from build123d import *

# Parameters (mm, degrees)
BOSS_EXTRUDE1_DEPTH = 16
SKETCH2_W           = 1.5
SKETCH2_H           = 16
BOSS_EXTRUDE2_DEPTH = 0.8
SKETCH3_W           = 16.5
SKETCH3_H           = 16
BOSS_EXTRUDE3_DEPTH = 20.8
SKETCH4_W           = 24.15
SKETCH4_H           = 16
BOSS_EXTRUDE4_DEPTH = 3.5
CUT_EXTRUDE1_DEPTH  = 6.5
CUT_EXTRUDE2_DEPTH  = 2
CUT_EXTRUDE3_DEPTH  = 2
SKETCH8_W           = 3
SKETCH8_H           = 7
CUT_EXTRUDE4_DEPTH  = 2.5
CUT_EXTRUDE5_DEPTH  = 1
SKETCH10_W          = 3.5
SKETCH10_H          = 16
BOSS_EXTRUDE5_DEPTH = 1.85
SKETCH11_W          = 2
SKETCH11_H          = 16.5
CUT_EXTRUDE6_DEPTH  = 9.8
SKETCH12_W          = 16.5
SKETCH12_H          = 1
CUT_EXTRUDE7_DEPTH  = 5.5
BOSS_EXTRUDE6_DEPTH = 7.5
CUT_EXTRUDE8_DEPTH  = 7.5
CUT_EXTRUDE9_DEPTH  = 7.5
SKETCH16_W          = 0.6
SKETCH16_H          = 7
BOSS_EXTRUDE7_DEPTH = 8
SKETCH17_W          = 6.5
SKETCH17_H          = 1.1
CUT_EXTRUDE10_DEPTH = 33.205641493
SKETCH18_W          = 6.5
SKETCH18_H          = 1.1
CUT_EXTRUDE11_DEPTH = 33.205641493
SKETCH19_W          = 0.6
SKETCH19_H          = 7
BOSS_EXTRUDE8_DEPTH = 8
SKETCH20_W          = 6.5
SKETCH20_H          = 1.1
CUT_EXTRUDE12_DEPTH = 32.849473214
SKETCH21_W          = 6.5
SKETCH21_H          = 1.1
CUT_EXTRUDE13_DEPTH = 32.849473214
CUT_EXTRUDE14_REACH = 33.068
CUT_EXTRUDE15_REACH = 34.206
CUT_EXTRUDE16_DEPTH = 32.849473214
CUT_EXTRUDE17_DEPTH = 7.5
CUT_EXTRUDE18_DEPTH = 1.5
CUT_EXTRUDE19_DEPTH = 1.5
SKETCH28_W          = 1.524
SKETCH28_H          = 7.988
CUT_EXTRUDE20_DEPTH = 18
SKETCH29_W          = 1.524
SKETCH29_H          = 6.35
CUT_EXTRUDE21_DEPTH = 18
CHAMFER1_SIZE       = 0.5
CHAMFER2_SIZE       = 0.528136002
CHAMFER2_SIZE2      = 0.608008164
CHAMFER3_SIZE       = 0.4
CHAMFER3_SIZE2      = 0.692820323
CHAMFER4_SIZE       = 0.608008164
CHAMFER4_SIZE2      = 0.528136002
CHAMFER5_SIZE       = 1.5
CHAMFER5_SIZE2      = 2.598076211


with BuildPart() as part:
    # Sketch1 → Boss-Extrude1 (new body)
    with BuildSketch(Plane.XZ.offset(8)):
        Polygon((12.803267754, -0.8), (9.65, -0.8), (9.65, -14.690909091), (10.15, -11.6), (10.15, -8.6), align=None)
    extrude(amount=-BOSS_EXTRUDE1_DEPTH)

    # Sketch2 → Boss-Extrude2 (add)
    with BuildSketch(Plane.XY.offset(-0.8)):
        with Locations((10.4, 0)):
            Rectangle(SKETCH2_W, SKETCH2_H)
    extrude(amount=BOSS_EXTRUDE2_DEPTH)

    # Sketch3 → Boss-Extrude3 (add)
    with BuildSketch(Plane.ZY.offset(-9.65)):
        with Locations((-8.25, 0)):
            Rectangle(SKETCH3_W, SKETCH3_H)
    extrude(amount=BOSS_EXTRUDE3_DEPTH)

    # Sketch4 → Boss-Extrude4 (add)
    with BuildSketch(Plane.XY):
        with Locations((0.925, 0)):
            Rectangle(SKETCH4_W, SKETCH4_H)
    extrude(amount=BOSS_EXTRUDE4_DEPTH)

    # Sketch5 → Cut-Extrude1 (cut)
    with BuildSketch(Plane(origin=(0, 8, 0), x_dir=(-1, 0, 0), z_dir=(0, 1, 0))):
        Polygon((-9.65, -14.690909091), (-9.65, -6.5), (-11.15, -3.5), (-11.15, -0.8), (-12.803267754, -0.8), (-10.15, -8.6), (-10.15, -11.6), align=None)
    extrude(amount=-CUT_EXTRUDE1_DEPTH, mode=Mode.SUBTRACT)

    # Sketch6 → Cut-Extrude2 (cut)
    with BuildSketch(Plane(origin=(0, 8, 0), x_dir=(-1, 0, 0), z_dir=(0, 1, 0))):
        Polygon((-11.15, 0), (-11.15, -3.5), (-9.65, -6.5), (-9.65, -16.5), (11.15, -16.5), (11.15, 0), align=None)
    extrude(amount=-CUT_EXTRUDE2_DEPTH, mode=Mode.SUBTRACT)

    # Sketch7 → Cut-Extrude3 (cut)
    with BuildSketch(Plane.XZ.offset(8)):
        Polygon((11.15, -0.8), (11.15, 0), (-11.15, 0), (-11.15, -16.5), (9.65, -16.5), (9.65, -14.690909091), (10.15, -11.6), (10.15, -8.6), (12.803267754, -0.8), align=None)
    extrude(amount=-CUT_EXTRUDE3_DEPTH, mode=Mode.SUBTRACT)

    # Sketch8 → Cut-Extrude4 (cut)
    with BuildSketch(Plane.XZ.offset(6)):
        with Locations((0, -3.5)):
            Rectangle(SKETCH8_W, SKETCH8_H)
    extrude(amount=-CUT_EXTRUDE4_DEPTH, mode=Mode.SUBTRACT)

    # Sketch9 → Cut-Extrude5 (cut)
    with BuildSketch(Plane.XZ.offset(6)):
        Polygon((-1.5, -7), (-1.5, -16.5), (7, -16.5), (7, 0), (1.5, 0), (1.5, -7), align=None)
    extrude(amount=-CUT_EXTRUDE5_DEPTH, mode=Mode.SUBTRACT)

    # Sketch10 → Boss-Extrude5 (add)
    with BuildSketch(Plane.ZY.offset(11.15)):
        with Locations((1.75, 0)):
            Rectangle(SKETCH10_W, SKETCH10_H)
    extrude(amount=BOSS_EXTRUDE5_DEPTH)

    # Sketch11 → Cut-Extrude6 (cut)
    with BuildSketch(Plane.XZ.offset(6)):
        with Locations((-10.15, -8.25)):
            Rectangle(SKETCH11_W, SKETCH11_H)
    extrude(amount=-CUT_EXTRUDE6_DEPTH, mode=Mode.SUBTRACT)

    # Sketch12 → Cut-Extrude7 (cut)
    with BuildSketch(Plane(origin=(-1.5, 0, 0), x_dir=(0, 0, -1), z_dir=(1, 0, 0))):
        with Locations((8.25, -5.5)):
            Rectangle(SKETCH12_W, SKETCH12_H)
    extrude(amount=-CUT_EXTRUDE7_DEPTH, mode=Mode.SUBTRACT)

    # Sketch13 → Boss-Extrude6 (add)
    with BuildSketch(Plane.XZ.offset(6)):
        Polygon((-9.15, -6.566987298), (-10.695259589, -0.8), (-12.803267754, -0.8), (-10.15, -8.6), (-10.15, -11.6), (-9.6, -15), (-9.6, -16.5), (-9.15, -16.5), align=None)
    extrude(amount=-BOSS_EXTRUDE6_DEPTH)

    # Sketch14 → Cut-Extrude8 (cut)
    with BuildSketch(Plane.XZ.offset(6)):
        with BuildLine():
            Line((-9.15, 0), (-9.15, -6.566987298))
            Line((-9.15, -6.566987298), (-8.9, -7.5))
            Line((-8.9, -7.5), (-8.9, -9.5))
            ThreePointArc((-8.9, -9.5), (-8.45, -9.95), (-8, -9.5))
            Line((-8, -9.5), (-8, 0))
            Line((-8, 0), (-9.15, 0))
        make_face()
    extrude(amount=-CUT_EXTRUDE8_DEPTH, mode=Mode.SUBTRACT)

    # Sketch15 → Cut-Extrude9 (cut)
    with BuildSketch(Plane.XZ.offset(6)):
        with BuildLine():
            Line((8.9, -9.5), (8.9, -7.5))
            Line((8.9, -7.5), (10.695259589, -0.8))
            Line((10.695259589, -0.8), (11.15, -0.8))
            Line((11.15, -0.8), (11.15, 0))
            Line((11.15, 0), (8, 0))
            Line((8, 0), (8, -9.5))
            ThreePointArc((8, -9.5), (8.45, -9.95), (8.9, -9.5))
        make_face()
    extrude(amount=-CUT_EXTRUDE9_DEPTH, mode=Mode.SUBTRACT)

    # Sketch16 → Boss-Extrude7 (add)
    with BuildSketch(Plane(origin=(0, 0, -16.5), x_dir=(-1, 0, 0), z_dir=(0, 0, -1))):
        with Locations((-6.012, 0)):
            Rectangle(SKETCH16_W, SKETCH16_H)
    extrude(amount=BOSS_EXTRUDE7_DEPTH)

    # Sketch17 → Cut-Extrude10 (cut, through all)
    with BuildSketch(Plane(origin=(6.312, 0, 0), x_dir=(0, 0, -1), z_dir=(1, 0, 0))):
        with Locations((21.25, 2.95)):
            Rectangle(SKETCH17_W, SKETCH17_H)
    extrude(amount=-CUT_EXTRUDE10_DEPTH, mode=Mode.SUBTRACT)

    # Sketch18 → Cut-Extrude11 (cut, through all)
    with BuildSketch(Plane(origin=(6.312, 0, 0), x_dir=(0, 0, -1), z_dir=(1, 0, 0))):
        with Locations((21.25, -2.95)):
            Rectangle(SKETCH18_W, SKETCH18_H)
    extrude(amount=-CUT_EXTRUDE11_DEPTH, mode=Mode.SUBTRACT)

    # Sketch19 → Boss-Extrude8 (add)
    with BuildSketch(Plane(origin=(0, 0, -16.5), x_dir=(-1, 0, 0), z_dir=(0, 0, -1))):
        with Locations((6.012, 0)):
            Rectangle(SKETCH19_W, SKETCH19_H)
    extrude(amount=BOSS_EXTRUDE8_DEPTH)

    # Sketch20 → Cut-Extrude12 (cut, through all)
    with BuildSketch(Plane(origin=(-5.712, 0, 0), x_dir=(0, 0, -1), z_dir=(1, 0, 0))):
        with Locations((21.25, 2.95)):
            Rectangle(SKETCH20_W, SKETCH20_H)
    extrude(amount=-CUT_EXTRUDE12_DEPTH, mode=Mode.SUBTRACT)

    # Sketch21 → Cut-Extrude13 (cut, through all)
    with BuildSketch(Plane(origin=(-5.712, 0, 0), x_dir=(0, 0, -1), z_dir=(1, 0, 0))):
        with Locations((21.25, -2.95)):
            Rectangle(SKETCH21_W, SKETCH21_H)
    extrude(amount=-CUT_EXTRUDE13_DEPTH, mode=Mode.SUBTRACT)

    # Sketch22 → Cut-Extrude14 (cut, up to next)
    with BuildSketch(Plane(origin=(0, 6, 0), x_dir=(-1, 0, 0), z_dir=(0, 1, 0)), mode=Mode.PRIVATE) as cut_extrude14_sk1:
        Polygon((11.15, -3.5), (9.65, -6.5), (9.65, -16.5), (11.15, -16.5), align=None)
    cut_extrude14_tool1 = extrude(cut_extrude14_sk1.sketch, amount=-CUT_EXTRUDE14_REACH, mode=Mode.PRIVATE) & part.part
    add(cut_extrude14_tool1.solids().sort_by_distance((-10.432609, 6, -10.717391))[0], mode=Mode.SUBTRACT)

    # Sketch23 → Cut-Extrude15 (cut, up to next)
    with BuildSketch(Plane(origin=(6.312, 0, 0), x_dir=(0, 0, -1), z_dir=(1, 0, 0)), mode=Mode.PRIVATE) as cut_extrude15_sk1:
        with BuildLine():
            Line((20, -1.4), (21.2, -1.4))
            ThreePointArc((21.2, -1.4), (22.6, 0), (21.2, 1.4))
            Line((21.2, 1.4), (20, 1.4))
            ThreePointArc((20, 1.4), (18.6, 0), (20, -1.4))
        make_face()
    cut_extrude15_tool1 = extrude(cut_extrude15_sk1.sketch, amount=-CUT_EXTRUDE15_REACH, mode=Mode.PRIVATE) & part.part
    add(cut_extrude15_tool1.solids().sort_by_distance((6.312, 0, -20.6))[0], mode=Mode.SUBTRACT)

    # Sketch24 → Cut-Extrude16 (cut, through all)
    with BuildSketch(Plane(origin=(-5.712, 0, 0), x_dir=(0, 0, -1), z_dir=(1, 0, 0))):
        with BuildLine():
            Line((20, -1.4), (21.2, -1.4))
            ThreePointArc((21.2, -1.4), (22.6, 0), (21.2, 1.4))
            Line((21.2, 1.4), (20, 1.4))
            ThreePointArc((20, 1.4), (18.6, 0), (20, -1.4))
        make_face()
    extrude(amount=-CUT_EXTRUDE16_DEPTH, mode=Mode.SUBTRACT)

    # Sketch25 → Cut-Extrude17 (cut)
    with BuildSketch(Plane.XZ.offset(6)):
        Polygon((9.6, -15), (9.6, -16.5), (9.65, -16.5), (9.65, -14.690909091), align=None)
    extrude(amount=-CUT_EXTRUDE17_DEPTH, mode=Mode.SUBTRACT)

    # Sketch26 → Cut-Extrude18 (cut)
    with BuildSketch(Plane.XZ.offset(5)):
        Polygon((2.2, -13.5), (3.191, -13.5), (3.191, -8.5), (1, -8.5), (1, -12.7), (2.2, -12.7), align=None)
    extrude(amount=-CUT_EXTRUDE18_DEPTH, mode=Mode.SUBTRACT)

    # Sketch27 → Cut-Extrude19 (cut)
    with BuildSketch(Plane.XZ.offset(5)):
        Polygon((-2.2, -13.5), (-2.2, -12.7), (-1, -12.7), (-1, -8.5), (-3.191, -8.5), (-3.191, -13.5), align=None)
    extrude(amount=-CUT_EXTRUDE19_DEPTH, mode=Mode.SUBTRACT)

    # Sketch28 → Cut-Extrude20 (cut)
    with BuildSketch(Plane.XY.offset(3.5)):
        with Locations((-6.35, 0)):
            Rectangle(SKETCH28_W, SKETCH28_H)
    extrude(amount=-CUT_EXTRUDE20_DEPTH, mode=Mode.SUBTRACT)

    # Sketch29 → Cut-Extrude21 (cut)
    with BuildSketch(Plane.XY.offset(3.5)):
        with Locations((6.35, 0)):
            Rectangle(SKETCH29_W, SKETCH29_H)
    extrude(amount=-CUT_EXTRUDE21_DEPTH, mode=Mode.SUBTRACT)

    # Chamfer1
    chamfer1_edges = [part.edges().sort_by_distance(p)[0] for p in [
        (6.012, 2.4, -24.5),
        (6.012, -2.4, -24.5),
        (-6.012, 2.4, -24.5),
        (-6.012, -2.4, -24.5),
    ]]
    chamfer(chamfer1_edges, length=CHAMFER1_SIZE)

    # Chamfer2
    chamfer2_edges = [part.edges().sort_by_distance(p)[0] for p in [
        (-12.803267754, -2.25, -0.8),
    ]]
    chamfer2_side = [part.faces().sort_by_distance(p)[0] for p in [
        (-11.476633877, -2.25, -4.7),
    ]]
    chamfer(chamfer2_edges, length=CHAMFER2_SIZE, length2=CHAMFER2_SIZE2, reference=chamfer2_side[0])

    # Chamfer3
    chamfer3_edges = [part.edges().sort_by_distance(p)[0] for p in [
        (-6.35, -3.994, 3.5),
        (-5.588, 0, 3.5),
        (-6.35, 3.994, 3.5),
        (-7.112, 0, 3.5),
        (6.35, -3.175, 3.5),
        (7.112, 0, 3.5),
        (6.35, 3.175, 3.5),
        (5.588, 0, 3.5),
    ]]
    chamfer3_side = [part.faces().sort_by_distance(p)[0] for p in [
        (0.040217242, 0, 3.5),
    ]]
    chamfer(chamfer3_edges, length=CHAMFER3_SIZE, length2=CHAMFER3_SIZE2, reference=chamfer3_side[0])

    # Chamfer4
    chamfer4_edges = [part.edges().sort_by_distance(p)[0] for p in [
        (12.803267754, -2.25, -0.8),
    ]]
    chamfer4_side = [part.faces().sort_by_distance(p)[0] for p in [
        (11.749263671, -2.25, -0.8),
    ]]
    chamfer(chamfer4_edges, length=CHAMFER4_SIZE, length2=CHAMFER4_SIZE2, reference=chamfer4_side[0])

    # Chamfer5
    chamfer5_edges = [part.edges().sort_by_distance(p)[0] for p in [
        (-13, 0, 3.5),
        (0, -8, 3.5),
        (13, 0, 3.5),
        (0, 8, 3.5),
    ]]
    chamfer5_side = [part.faces().sort_by_distance(p)[0] for p in [
        (0.06378672, 0, 3.5),
    ]]
    chamfer(chamfer5_edges, length=CHAMFER5_SIZE, length2=CHAMFER5_SIZE2, reference=chamfer5_side[0])


solid = part.part
The model under review builds one solid part; all positions refer to its coordinate system, in mm. A direction names the side the tool comes from. Coordinates: 2 decimals unless noted, no trailing zeros. Loops run counter-clockwise (first coordinate to the right, second up) from the corner with the lowest first, then second, coordinate; pieces in that order, holes last. Notation, with made-up numbers: (-32, 59.5) -> (21, 59.5) arc R25 cw to (21, 76.5) -> close; hole circle Ø11 at (-5.5, 22.5). An arc over 180 degrees is marked (long way). Use a Markdown table: item, result. Add a question column.
1. Clearance check with flat-ended pins moving along their axes: pin 1 Ø1 at (x, z) = (-6.5, -13) entering from +Y; pin 2 Ø1.2 at (y, z) = (-4.5, -10.5) entering from -X; pin 3 Ø1.6 at (y, z) = (-4, -5) entering from +X. State where each tip first meets the part, or that it passes through.
2. Machinability: for faces 5 (the face through (5.588, 0, -6)), 6 (the face through (9.6, -2, -16)), 7 (the face through (10.15, -2, -10)), 8 (the face through (0, 6, -8)), 9 (the face through (-8.9, -2, -8)), which of the approach directions +Z, -Z, +X, -X, +Y, -Y give a long, thin tool a straight path to every point of the face, cutting with its end or side? Answer none if there is none.
3. To check wall thickness, follow line 1 (X direction, y = -2.25, z = -18.5); line 2 (X direction, y = -1.5, z = -11.25); line 3 (Y direction, x = 6.25, z = -20.5). State the ranges of each line that lie inside material, in increasing order.
4. Add section C-C on x = 8.45. Write out the cut boundary in (y, z).
5. Add section B-B on x = 3.75. Write out the cut boundary in (y, z).
6. Draft analysis for pull direction Z (two halves, no side actions). For faces 1 (the face through (2, -4, -8.5)), 2 (the face through (0, -3.5, -3)), 3 (the face through (6.312, -2, -20)), 4 (the face through (-12.26, -0.11, 2.18)), state which applies: pulls with the +Z half, pulls with the -Z half, needs draft (parallel to the pull), parting line crosses it, or undercut.
7. Add section A-A on y = 0. Give the number of separate pieces and of enclosed holes in the cut face, plus the area to 3 significant figures.
Returned:
| question | item | result |
|---|---|---|
| 1 | pin 1 | stops at y = 6 |
| 1 | pin 2 | stops at x = -10.15 |
| 1 | pin 3 | stops at x = 11.65 |
| 2 | face 5 | +Z |
| 2 | face 6 | -Z, +X, -Y |
| 2 | face 7 | -Z, +X, +Y, -Y |
| 2 | face 8 | -Z, +X, -X, +Y |
| 2 | face 9 | -Y |
| 3 | line 1 | x = -6.31 to -5.71, 5.71 to 6.31 |
| 3 | line 2 | x = -10.15 to -7.11, -5.59 to 5.59, 7.11 to 10.15 |
| 3 | line 3 | y = -2.4 to -1.4, 1.4 to 2.4 |
| 4 | outline | (-8, 0) -> (1.5, 0) -> (1.5, -9.95) -> (-6, -9.95) -> (-6, -16.5) -> (6, -16.5) -> (6, 0) -> (8, 0) -> (8, 0.9) -> (6.5, 3.5) -> (-6.5, 3.5) -> (-8, 0.9) -> close |
| 5 | outline | (-8, 0) -> (-5, 0) -> (-5, -16.5) -> (6, -16.5) -> (6, 0) -> (8, 0) -> (8, 0.9) -> (6.5, 3.5) -> (-6.5, 3.5) -> (-8, 0.9) -> close |
| 6 | face 1 | undercut |
| 6 | face 2 | undercut |
| 6 | face 3 | needs draft |
| 6 | face 4 | pulls with the +Z half |
| 7 | separate pieces | 3 |
| 7 | enclosed holes | 0 |
| 7 | area | 357 mm² |
